```python
from build123d import *

# Parameters (mm, degrees)
BOSS_EXTRUDE1_DEPTH  = 5
SKETCH2_R            = 4
CUT_EXTRUDE1_DEPTH   = 10
LPATTERN1_COUNT      = 2
LPATTERN1_PITCH      = 140
LPATTERN1_COUNT_DIR2 = 2
LPATTERN1_PITCH_DIR2 = 140
SKETCH3_R            = 50
BOSS_EXTRUDE2_DEPTH  = 20
SKETCH5_R            = 15
CUT_EXTRUDE3_DEPTH   = 50


with BuildPart() as part:
    # Sketch1 → Boss-Extrude1 (new body)
    with BuildSketch(Plane(origin=(0, 0, 0), x_dir=(1, 0, 0), z_dir=(0, 1, 0))):
        with BuildLine():
            Line((10, 0), (170, 0))
            ThreePointArc((170, 0), (177.071067812, 2.928932188), (180, 10))
            Line((180, 10), (180, 170))
            ThreePointArc((180, 170), (177.071067812, 177.071067812), (170, 180))
            Line((170, 180), (10, 180))
            ThreePointArc((10, 180), (2.928932188, 177.071067812), (0, 170))
            Line((0, 170), (0, 10))
            ThreePointArc((0, 10), (2.928932188, 2.928932188), (10, 0))
        make_face()
    extrude(amount=BOSS_EXTRUDE1_DEPTH)

    # Sketch2 → Cut-Extrude1 (cut)
    with BuildSketch(Plane(origin=(0, 5, 0), x_dir=(1, 0, 0), z_dir=(0, 1, 0))):
        with Locations(Location((20, 20, 0), (0, 0, 270))):
            Circle(SKETCH2_R)
    cut_extrude1 = extrude(amount=-CUT_EXTRUDE1_DEPTH, mode=Mode.SUBTRACT)

    # LPattern1: Cut-Extrude1 2 × 2
    with Locations(*[(i * LPATTERN1_PITCH, 0, -j * LPATTERN1_PITCH_DIR2) for i in range(LPATTERN1_COUNT) for j in range(LPATTERN1_COUNT_DIR2) if (i, j) != (0, 0)]):
        add(cut_extrude1, mode=Mode.SUBTRACT)

    # Sketch3 → Boss-Extrude2 (add)
    with BuildSketch(Plane(origin=(0, 5, 0), x_dir=(1, 0, 0), z_dir=(0, 1, 0))):
        with Locations(Location((90, 90, 0), (0, 0, 270))):
            Circle(SKETCH3_R)
    extrude(amount=BOSS_EXTRUDE2_DEPTH)

    # Sketch5 → Cut-Extrude3 (cut)
    with BuildSketch(Plane(origin=(0, 25, 0), x_dir=(1, 0, 0), z_dir=(0, 1, 0))):
        with Locations(Location((90, 90, 0), (0, 0, 270))):
            Circle(SKETCH5_R)
    extrude(amount=-CUT_EXTRUDE3_DEPTH, mode=Mode.SUBTRACT)


solid = part.part
```
Source: CAD feature listing. Evaluate the final solid. Frame: model axes, mm. A direction names the side the tool comes from. Coordinates: 2 decimals unless noted, no trailing zeros. Loops run counter-clockwise (first coordinate to the right, second up) from the corner with the lowest first, then second, coordinate; pieces in that order, holes last. Notation, with made-up numbers: M 23,18.5 L 75,18.5 A25 cw 75,48.5 Z; hole C 74,71 d11. An arc over 180 degrees is marked long. Put each result on its own line as item: value. Start each with the question number.
1) Pull-direction query (Z, two-part tool) for faces 1 (the face through (89, 2, 0)), 2 (the face through (0, 2, -91)), 3 (the face through (23.966, 2.535, -20.521)), 4 (the face through (163.373, 2.535, -157.85)); classes: pulls with the +Z half, pulls with the -Z half, needs draft (parallel to the pull), parting line crosses it, or undercut.
2) Cut plane C-C on x = 160. Return the cut outline in (y, z), then the cut area to 3 significant figures.
3) Ray query, L1, parallel to X at y = 1.6, z = -160; L2, parallel to X at y = 18.5, z = -90; L3, parallel to Y at x = 137, z = -34.5. Return the intervals inside material, ascending. Write a range as from..to.
4) Cut plane D-D on z = -90. Return the cut outline in (x, y), then the cut area to 3 significant figures.
5) Cut plane A-A on z = -160. Return the cut outline in (x, y), then the cut area to 3 significant figures.
6) Contact query for flat-ended pins moving along their axis: pin 1 Ø10.5 at (x, z) = (20, -20) entering from +Y; pin 2 Ø24 at (x, z) = (90, -90) entering from -Y. Output: stop coordinate, or through.
7) Cut plane B-B on x = 90. Return the cut outline in (y, z), then the cut area to 3 significant figures.
8) Reachability of faces 5 (the face through (41.19, 14.86, -100.84)), 6 (the face through (21.201, 2.535, -156.185)) from +Z, -Z, +X, -X, +Y, -Y: full face, straight path, thin tool, end or side. Return the list, or none.
The answers:
1. face 1: pulls with the +Z half
1. face 2: needs draft
1. face 3: undercut
1. face 4: undercut
2. outline: M 0,-180 L 5,-180 L 5,-164 L 0,-164 Z; M 0,-156 L 5,-156 L 5,-24 L 0,-24 Z; M 0,-16 L 5,-16 L 5,0 L 0,0 Z
2. area: 820 mm²
3. L1: x = 0..16, 24..156, 164..180
3. L2: x = 40..75, 105..140
3. L3: y = 0..5
4. outline: M 0,0 L 75,0 L 75,25 L 40,25 L 40,5 L 0,5 Z; M 105,0 L 180,0 L 180,5 L 140,5 L 140,25 L 105,25 Z
4. area: 2,150 mm²
5. outline: M 0,0 L 16,0 L 16,5 L 0,5 Z; M 24,0 L 156,0 L 156,5 L 24,5 Z; M 164,0 L 180,0 L 180,5 L 164,5 Z
5. area: 820 mm²
6. pin 1: stops at y = 5
6. pin 2: passes through
7. outline: M 0,-180 L 5,-180 L 5,-140 L 25,-140 L 25,-105 L 0,-105 Z; M 0,-75 L 25,-75 L 25,-40 L 5,-40 L 5,0 L 0,0 Z
7. area: 2,150 mm²
8. face 5: +Y
8. face 6: +Y, -Y
